Study the drawing (mm; zero at the part's minimum x, y, z) and answer. Round coordinates to 2 decimals unless told otherwise and drop trailing zeros. Order: outer loops, then holes, each group sorted by start corner. A loop starts at its lowest first (then second) coordinate and runs counter-clockwise, first axis right, second up. Notation, with made-up numbers: (54.5, 24) - (108.5, 24) arc R13 cw to (108.5, 38) - close; hole circle Ø11 at (72.25, 24.5). An arc over 180 degrees is marked (long way). Put each result on its own line as item: value.
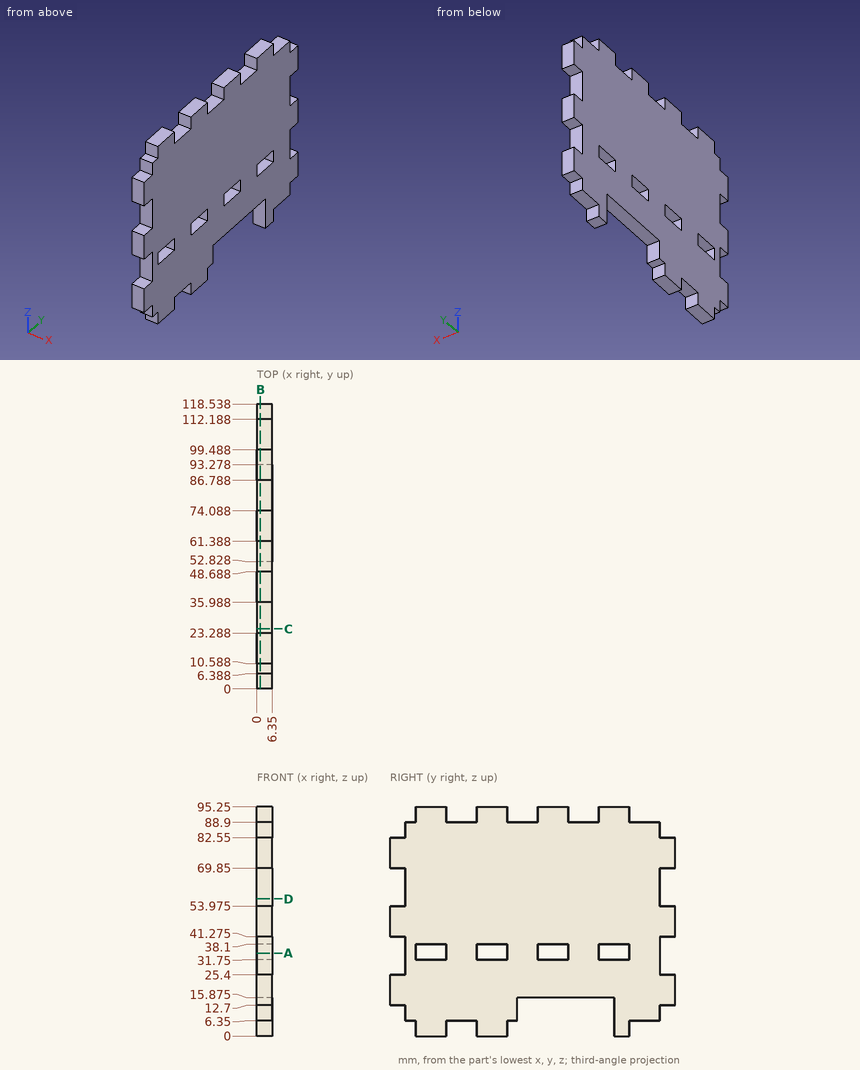
1) Given pin 1 Ø1.5 at (x, y) = (2, 28.5) entering from -Z; pin 2 Ø3 at (x, y) = (3.5, 115.5) entering from -Z; pin 3 Ø1 at (y, z) = (75, 79.5) entering from -X; pin 4 Ø1.9 at (x, z) = (4, 4) entering from -Y, each flat-ended and moving along its own axis, determine where each tip first touches the part or whether it passes through.
Findings below:
pin 1: stops at z = 6.35
pin 2: stops at z = 12.7
pin 3: stops at x = 0
pin 4: stops at y = 10.59
2) A cutting plane is placed at B-B on x = 1.5. Give the number of separate pieces and of enclosed holes in the cut face.
Findings below:
separate pieces: 1
enclosed holes: 4
3) A cutting plane is placed at A-A on z = 34.5. Write down the section's boundary in (x, y).
Findings below:
outline: (0, 6.39) - (6.35, 6.39) - (6.35, 10.59) - (0, 10.59) - close; (0, 23.29) - (6.35, 23.29) - (6.35, 35.99) - (0, 35.99) - close; (0, 48.69) - (6.35, 48.69) - (6.35, 61.39) - (0, 61.39) - close; (0, 74.09) - (6.35, 74.09) - (6.35, 86.79) - (0, 86.79) - close; (0, 99.49) - (6.35, 99.49) - (6.35, 112.19) - (0, 112.19) - close
4) A cutting plane is placed at C-C on y = 25. Write down the section's boundary in (x, z).
Findings below:
outline: (0, 6.35) - (6.35, 6.35) - (6.35, 88.9) - (0, 88.9) - close
5) A cutting plane is placed at D-D on z = 57. Write down the section's boundary in (x, y), then the cut area to 3 significant figures.
Findings below:
outline: (0, 6.39) - (6.35, 6.39) - (6.35, 112.19) - (0, 112.19) - close
area: 672 mm2
6) Straight lines are drawn through the part: L1, parallel to Y at x = 0.75, z = 35; L2, parallel to Y at x = 4.25, z = 11; L3, parallel to Z at x = 5.25, y = 38.5. For each, find the intervals that lie inside material, in ascending order. Write a range as from..to.
Findings below:
L1: y = 6.39..10.59, 23.29..35.99, 48.69..61.39, 74.09..86.79, 99.49..112.19
L2: y = 6.39..52.83, 93.28..112.19
L3: z = 0..31.75, 38.1..95.25
